The listing builds one solid part. Answer for the finished solid, in the listing's coordinates (mm). Coordinates: 2 decimals unless noted, no trailing zeros. Write each loop counter-clockwise with the first axis right and the second up, starting at its lowest first coordinate (ties: lowest second). Pieces come first, ordered by that corner, then holes.
from build123d import *

# Parameters (mm, degrees)
F0_R         = 5.2
F0_R_2       = 11
F1_DEPTH     = 8
F2_T2_ANGLE  = 163.5880718536
F2_T4_ANGLE  = 163.5880718536
F2_T6_ANGLE  = 163.5880718536
F2_T8_ANGLE  = 163.5880718536
F2_T10_ANGLE = 163.5880718536
F2_T12_ANGLE = 163.5880718536


# Not quite as in the source:
# - a fillet or chamfer that OpenCascade refuses, or shapes differently, is made with other operations: its cross-section is extruded or revolved along the edge and cut away or added


with BuildPart() as f1:
    # F0 (on Top) → F1 (new body)
    with BuildSketch(Plane.XY):
        with BuildLine():
            Line((10, 28.4363744997), (0, 45.7568825754))
            Line((0, 45.7568825754), (-10, 28.4363744997))
            ThreePointArc((-10, 28.4363744997), (-11.3397459622, 6.115866424), (-30, -6.2046416517))
            Line((-30, -6.2046416517), (-40, -23.5251497274))
            Line((-40, -23.5251497274), (-20, -23.5251497274))
            ThreePointArc((-20, -23.5251497274), (0, -13.5251497274), (20, -23.5251497274))
            Line((20, -23.5251497274), (40, -23.5251497274))
            Line((40, -23.5251497274), (30, -6.2046416517))
            ThreePointArc((30, -6.2046416517), (11.3397459622, 6.115866424), (10, 28.4363744997))
        make_face()
        with Locations((-25.2775681357, -15.0251497274)):
            Circle(F0_R, mode=Mode.SUBTRACT)
        with Locations((25.2775681357, -15.0251497274)):
            Circle(F0_R, mode=Mode.SUBTRACT)
        with Locations((0, -0.4311389598)):
            Circle(F0_R_2, mode=Mode.SUBTRACT)
        with Locations((0, 28.7568825754)):
            Circle(F0_R, mode=Mode.SUBTRACT)
    extrude(amount=F1_DEPTH)

    # F2: fillet of radius 5 on 6 edges, made by hand

    # F2_s1 → F2_t2 (revolve, cut)
    with BuildSketch(Plane(origin=(-29.4179701652, 23.1546186531, 0), x_dir=(0, 0, 1), z_dir=(-0.7857925171, 0.618490194, 0))):
        with BuildLine():
            ThreePointArc((3, 19.2239813561), (6.5355339059, 20.6884474501), (8, 24.2239813561))
            Line((8, 24.2239813561), (8, 19.2239813561))
            Line((8, 19.2239813561), (3, 19.2239813561))
        make_face()
    revolve(axis=Axis((-32.9903810568, 18.615866424, 8), (0, 0, -1)), revolution_arc=F2_T2_ANGLE, mode=Mode.SUBTRACT)

    # F2_s3 → F2_t4 (revolve, cut)
    with BuildSketch(Plane(origin=(34.8604405257, 13.9389723807, 0), x_dir=(0, 0, 1), z_dir=(0.9285244785, 0.3712711849, 0))):
        with BuildLine():
            ThreePointArc((3, 19.9630902024), (6.5355339059, 21.4275562964), (8, 24.9630902024))
            Line((8, 24.9630902024), (8, 19.9630902024))
            Line((8, 19.9630902024), (3, 19.9630902024))
        make_face()
    revolve(axis=Axis((32.9903810568, 18.615866424, 8), (0, 0, -1)), revolution_arc=F2_T4_ANGLE, mode=Mode.SUBTRACT)

    # F2_s5 → F2_t6 (revolve, cut)
    with BuildSketch(Plane(origin=(-5.4424703605, -37.7402994735, 0), x_dir=(0, 0, 1), z_dir=(-0.1427319614, -0.9897613789, 0))):
        with BuildLine():
            ThreePointArc((3, 19.5012298151), (6.5355339059, 20.9656959092), (8, 24.5012298151))
            Line((8, 24.5012298151), (8, 19.5012298151))
            Line((8, 19.5012298151), (3, 19.5012298151))
        make_face()
    revolve(axis=Axis((0, -38.5251497274, 8), (0, 0, -1)), revolution_arc=F2_T6_ANGLE, mode=Mode.SUBTRACT)

    # F2_s7 → F2_t8 (revolve, cut)
    with BuildSketch(Plane(origin=(-29.4179701652, 23.1546186531, 0), x_dir=(0, 0, 1), z_dir=(-0.7857925171, 0.618490194, 0))):
        with BuildLine():
            ThreePointArc((5, 19.2239813561), (1.4644660941, 20.6884474501), (0, 24.2239813561))
            Line((0, 24.2239813561), (0, 19.2239813561))
            Line((0, 19.2239813561), (5, 19.2239813561))
        make_face()
    revolve(axis=Axis((-32.9903810568, 18.615866424, 0), (0, 0, -1)), revolution_arc=F2_T8_ANGLE, mode=Mode.SUBTRACT)

    # F2_s9 → F2_t10 (revolve, cut)
    with BuildSketch(Plane(origin=(34.8604405257, 13.9389723807, 0), x_dir=(0, 0, 1), z_dir=(0.9285244785, 0.3712711849, 0))):
        with BuildLine():
            ThreePointArc((5, 19.9630902024), (1.4644660941, 21.4275562964), (0, 24.9630902024))
            Line((0, 24.9630902024), (0, 19.9630902024))
            Line((0, 19.9630902024), (5, 19.9630902024))
        make_face()
    revolve(axis=Axis((32.9903810568, 18.615866424, 0), (0, 0, -1)), revolution_arc=F2_T10_ANGLE, mode=Mode.SUBTRACT)

    # F2_s11 → F2_t12 (revolve, cut)
    with BuildSketch(Plane(origin=(-5.4424703605, -37.7402994735, 0), x_dir=(0, 0, 1), z_dir=(-0.1427319614, -0.9897613789, 0))):
        with BuildLine():
            ThreePointArc((5, 19.5012298151), (1.4644660941, 20.9656959092), (0, 24.5012298151))
            Line((0, 24.5012298151), (0, 19.5012298151))
            Line((0, 19.5012298151), (5, 19.5012298151))
        make_face()
    revolve(axis=Axis((0, -38.5251497274, 0), (0, 0, -1)), revolution_arc=F2_T12_ANGLE, mode=Mode.SUBTRACT)


solid = f1.part
1. Section C-C on y = 40.5 is taken. Give the vertices of the cut face in (x, z), then the cut area to 3 significant figures.
Results found:
outline: (-3.04, 0) - (3.04, 0) - (3.04, 8) - (-3.04, 8) - close
area: 48.6 mm2
2. Flat-ended cylindrical pins translate along their axes: P1, Ø3, axis at x = -4.5, y = 27.5, coming from the +Z side; P2, Ø1, axis at y = -8.5, z = 3, coming from the -X side; P3, Ø1, axis at x = 4, y = 20.5, coming from the -Z side. Find the tip coordinate at first contact, or state that the pin passes through.
Results found:
P1: stops at z = 7.98
P2: stops at x = -31.61
P3: stops at z = 0.02
3. Section A-A on z = 5 is taken. Give the vertices of the cut face in (x, y).
Results found:
outline: (-40, -23.53) - (-20.52, -23.53) arc R25.42 cw to (20.52, -23.53) - (40, -23.53) - (30.26, -6.65) arc R25.42 cw to (9.74, 28.89) - (0, 45.76) - (-9.74, 28.89) arc R25.42 cw to (-30.26, -6.65) - close; hole circle Ø10.4 at (-25.28, -15.03); hole circle Ø22 at (0, -0.43); hole circle Ø10.4 at (0, 28.76); hole circle Ø10.4 at (25.28, -15.03)
4. For a pull along Y with two mould halves and no side action, classify faces 1 (the flat face through (15, -9, 8)), 2 (the cylindrical face through (-1.13, 23.68, 3.94)), 3 (the flat face through (-30, -23.525, 4)) as pulls with the +Y half, pulls with the -Y half, needs draft (parallel to the pull), parting line crosses it, or undercut.
Results found:
face 1: needs draft
face 2: undercut
face 3: pulls with the -Y half
5. Find the intervals of material crossed by L1, parallel to Y at x = 4, z = 6.75; L2, parallel to X at y = -11.5, z = 5.5; L3, parallel to X at y = -4, z = 6, in increasing order.
Results found:
L1: y = -12.13 to -10.68, 9.82 to 25.43, 32.08 to 38.83
L2: x = -33.06 to -29.1, -21.45 to 21.45, 29.1 to 33.06
L3: x = -20.16 to -10.4, 10.4 to 20.16
6. Section B-B on y = -14 is taken. State how many separate pieces and enclosed holes the cut face has, then the cut area to 3 significant figures.
Results found:
separate pieces: 4
enclosed holes: 0
area: 242 mm2
